For this review, take the finished solid that the model builds, in its own axes (mm). A direction names the side the tool comes from. Coordinates: 2 decimals unless noted, no trailing zeros. Order: outer loops, then holes, each group sorted by start corner. A loop starts at its lowest first (then second) coordinate and runs counter-clockwise, first axis right, second up.
from build123d import *

# Parameters (mm, degrees)
BOSS_EXTRUDE1_DEPTH = 15
SKETCH2_R           = 1.6
SKETCH2_R_2         = 2.4
CUT_EXTRUDE1_DEPTH  = 22.847836945


with BuildPart() as part:
    # Sketch1 → Boss-Extrude1 (new body)
    with BuildSketch(Plane(origin=(0, 0, 0), x_dir=(1, 0, 0), z_dir=(0, 1, 0))):
        Polygon((0, 0), (10.25, 0), (12.75, 0), (12.75, 9.474464586), (9.25, 9.474464586), (1.5, 5), (0, 5), (-1.5, 5), (-9.25, 9.474464586), (-12.75, 9.474464586), (-12.75, 0), (-10.25, 0), align=None)
    extrude(amount=BOSS_EXTRUDE1_DEPTH)

    # Sketch2 → Cut-Extrude1 (cut, through all)
    with BuildSketch(Plane.XY):
        with Locations((-5.9, 12)):
            Circle(SKETCH2_R)
        with Locations((5.9, 12)):
            Circle(SKETCH2_R)
        with Locations((-7.625, 6)):
            Circle(SKETCH2_R_2)
        with Locations((7.625, 6)):
            Circle(SKETCH2_R_2)
    extrude(amount=-CUT_EXTRUDE1_DEPTH, mode=Mode.SUBTRACT)


solid = part.part
1. To check wall thickness, follow L1, parallel to X at y = 6, z = -2.25 (3 decimals); L2, parallel to X at y = 12, z = -4; L3, parallel to X at y = 12, z = -5.5. State the ranges of each line that lie inside material, in increasing order.
Answer below:
L1: x = -12.75 to -10.025, -5.225 to 5.225, 10.025 to 12.75
L2: x = -12.75 to -7.5, -4.3 to 4.3, 7.5 to 12.75
L3: x = -12.75 to -7.5, -4.3 to -2.37, 2.37 to 4.3, 7.5 to 12.75
2. Take a section at B-B, the plane y = 6. Give the boundary of the cut face in (x, z) (3 decimals).
Answer below:
outline: (-12.75, -9.474) - (-10.025, -9.474) - (-10.025, 0) - (-12.75, 0) - close; (-5.225, -7.151) - (-1.5, -5) - (1.5, -5) - (5.225, -7.151) - (5.225, 0) - (-5.225, 0) - close; (10.025, -9.474) - (12.75, -9.474) - (12.75, 0) - (10.025, 0) - close
3. Take a section at D-D, the plane z = -2. Give the boundary of the cut face in (x, y) (3 decimals), plus the area to 3 significant figures.
Answer below:
outline: (-12.75, 0) - (12.75, 0) - (12.75, 15) - (-12.75, 15) - close; hole circle Ø4.8 at (-7.625, 6); hole circle Ø3.2 at (-5.9, 12); hole circle Ø3.2 at (5.9, 12); hole circle Ø4.8 at (7.625, 6)
area: 330 mm2
4. Take a section at A-A, the plane z = -5.75. Give the boundary of the cut face in (x, y) (3 decimals).
Answer below:
outline: (-12.75, 0) - (-2.799, 0) - (-2.799, 15) - (-12.75, 15) - close; (2.799, 0) - (12.75, 0) - (12.75, 15) - (2.799, 15) - close; hole circle Ø4.8 at (-7.625, 6); hole circle Ø3.2 at (-5.9, 12); hole circle Ø3.2 at (5.9, 12); hole circle Ø4.8 at (7.625, 6)
5. Clearance check with flat-ended pins moving along their axes: pin 1 Ø3.5 at (x, y) = (5.9, 12) entering from -Z; pin 2 Ø2.5 at (x, y) = (0, 11) entering from -Z; pin 3 Ø1.5 at (x, y) = (-5, 4.5) entering from -Z. State where each tip first meets the part, or that it passes through.
Answer below:
pin 1: stops at z = -8.55
pin 2: stops at z = -5
pin 3: stops at z = -7.45
6. The part is to be moulded in two halves that separate along X. For faces 1 (the face through (-12.75, 7, -5)), 2 (the face through (0, 7, -5)), 3 (the face through (0, 15, -4)), say which applies: +X half, -X half, draft (parallel to the pull), parting line (faces both ways), or undercut.
Answer below:
face 1: -X half
face 2: undercut
face 3: draft
7. Machinability: for faces 4 (the face through (-4.46, 7.4, -6.71)), 5 (the face through (11, 7, -9.474)), which of the approach directions +Z, -Z, +X, -X, +Y, -Y give a long, thin tool a straight path to every point of the face, cutting with its end or side? Answer none if there is none.
Answer below:
face 4: -Z, +Y, -Y
face 5: -Z, +X, -X, +Y, -Y
8. Take a section at C-C, the plane x = 5.9. Give the boundary of the cut face in (y, z), plus the area to 3 significant figures.
Answer below:
outline: (0, -7.54) - (4.33, -7.54) - (4.33, 0) - (0, 0) - close; (7.67, -7.54) - (10.4, -7.54) - (10.4, 0) - (7.67, 0) - close; (13.6, -7.54) - (15, -7.54) - (15, 0) - (13.6, 0) - close
area: 63.8 mm2
